The figure shows three views and two pictorial views of one solid part (mm, origin at its lowest corner). Answer the questions. A direction names the side the tool comes from. Coordinates: 2 decimals unless noted, no trailing zeros. Write each loop counter-clockwise with the first axis right and the second up, starting at its lowest first coordinate (ties: lowest second). Pieces come first, ordered by that corner, then holes. Notation, with made-up numbers: (59.25, 48.5) -> (112.25, 48.5) arc R37 cw to (112.25, 86.5) -> close; hole circle Ø4 at (31.25, 77.5). An arc over 180 degrees is marked (long way). Use CSV: the item, a comma, the result in double quotes. Start each with the question number.
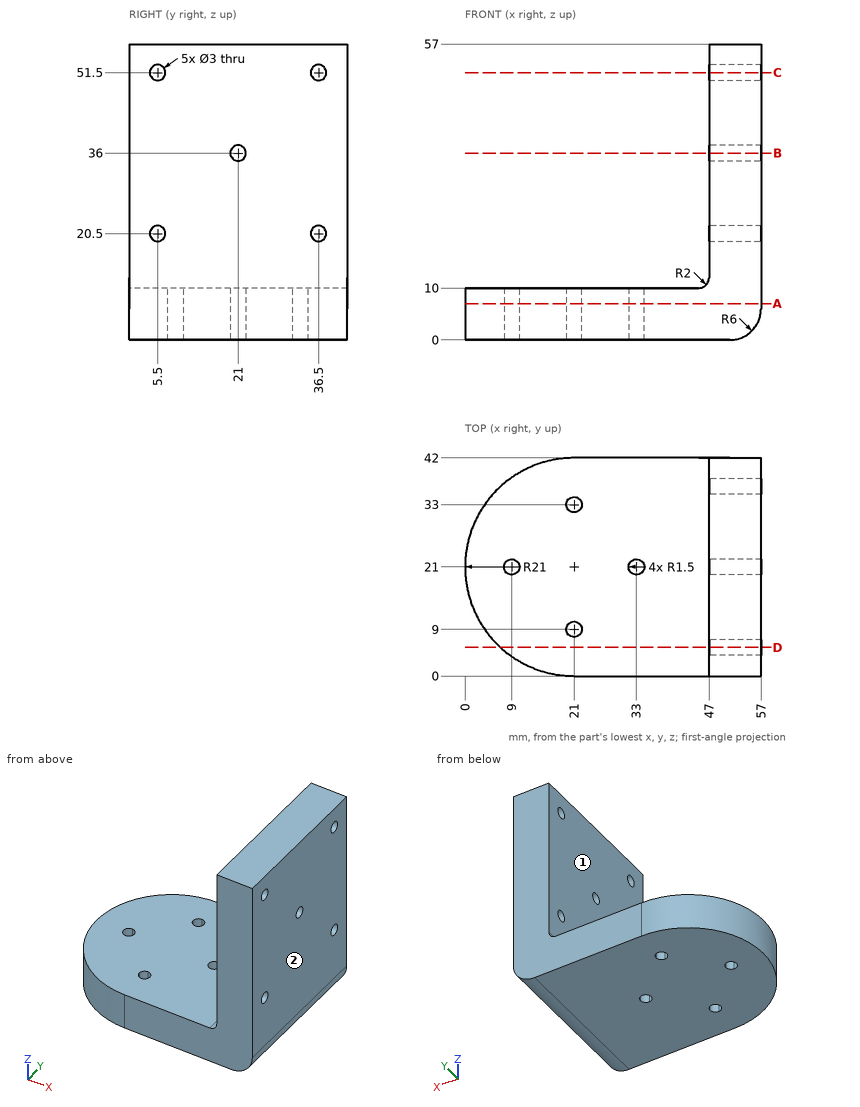
1) Which of the six approach directions +Z, -Z, +X, -X, +Y, -Y give full straight-line access (tool end or side, diameter ignored) to the marked faces 1 and 2?
2) Section C-C, the plane z = 51.5 is taken. Give the vertices of the cut face in (x, y).
3) Find the intervals of material crossed by line 1 along Y through (x, z) = (50.25, 20.5); line 2 along Y through (x, z) = (49.25, 36); line 3 along Z through (x, y) = (50, 36), in increasing order.
4) Each of these flat-tipped pins is pushed along its axis until it touches: pin 1 (2.5 mm diameter, centred on y = 36.5, z = 20.5, fed in from +X); pin 2 (12 mm diameter, centred on y = 22, z = 8.5, fed in from -X); pin 3 (12.5 mm diameter, centred on y = 17, z = 29.5, fed in from -X); pin 4 (2 mm diameter, centred on x = 32, y = 11.5, fed in from +Z). Where does it stop, or does it pass through?
5) Section A-A, the plane z = 7 is taken. Give the vertices of the cut face in (x, y), plus the area to 3 significant figures.
6) Section D-D, the plane y = 5.5 is taken. Give the vertices of the cut face in (x, z), plus the area to 3 significant figures.
7) Section B-B, the plane z = 36 is taken. Give the vertices of the cut face in (x, y), plus the area to 3 significant figures.
The answers:
1,face 1,"+Z, -X, +Y, -Y"
1,face 2,"+Z, -Z, +X, +Y, -Y"
2,outline,"(47, 0) -> (57, 0) -> (57, 4) -> (47, 4) -> close; (47, 7) -> (57, 7) -> (57, 35) -> (47, 35) -> close; (47, 38) -> (57, 38) -> (57, 42) -> (47, 42) -> close"
3,line 1,"y = 0 to 4, 7 to 35, 38 to 42"
3,line 2,"y = 0 to 19.5, 22.5 to 42"
3,line 3,"z = 0 to 19.09, 21.91 to 50.09, 52.91 to 57"
4,pin 1,"passes through"
4,pin 2,"stops at x = 0"
4,pin 3,"stops at x = 47"
4,pin 4,"stops at z = 10"
5,outline,"(21, 0) -> (57, 0) -> (57, 42) -> (21, 42) arc R21 ccw to start; hole circle Ø3 at (9, 21); hole circle Ø3 at (21, 9); hole circle Ø3 at (21, 33); hole circle Ø3 at (33, 21)"
5,area,"2,180 mm^2"
6,outline,"(6.83, 0) -> (51, 0) arc R6 ccw to (57, 6) -> (57, 19) -> (47, 19) -> (47, 12) arc R2 cw to (45, 10) -> (6.83, 10) -> close; (47, 22) -> (57, 22) -> (57, 50) -> (47, 50) -> close; (47, 53) -> (57, 53) -> (57, 57) -> (47, 57) -> close"
6,area,"905 mm^2"
7,outline,"(47, 0) -> (57, 0) -> (57, 19.5) -> (47, 19.5) -> close; (47, 22.5) -> (57, 22.5) -> (57, 42) -> (47, 42) -> close"
7,area,"390 mm^2"
